Geometry: see drawing. Coordinates: mm, zero at the bounding-box minimum. Give positions to 0.01 mm unless a question says otherwise; leave off trailing zeros. Order: outer loops, then holes, each group sorted by start corner. A loop starts at its lowest first (then second) coordinate and runs counter-clockwise, first axis right, second up. Notation, with made-up numbers: M 79.5,37.25 L 109.5,37.25 A22 cw 109.5,56.25 Z; hole C 1,67.5 d4. An arc over 180 degrees is marked long. Use a Markdown table: item, result.
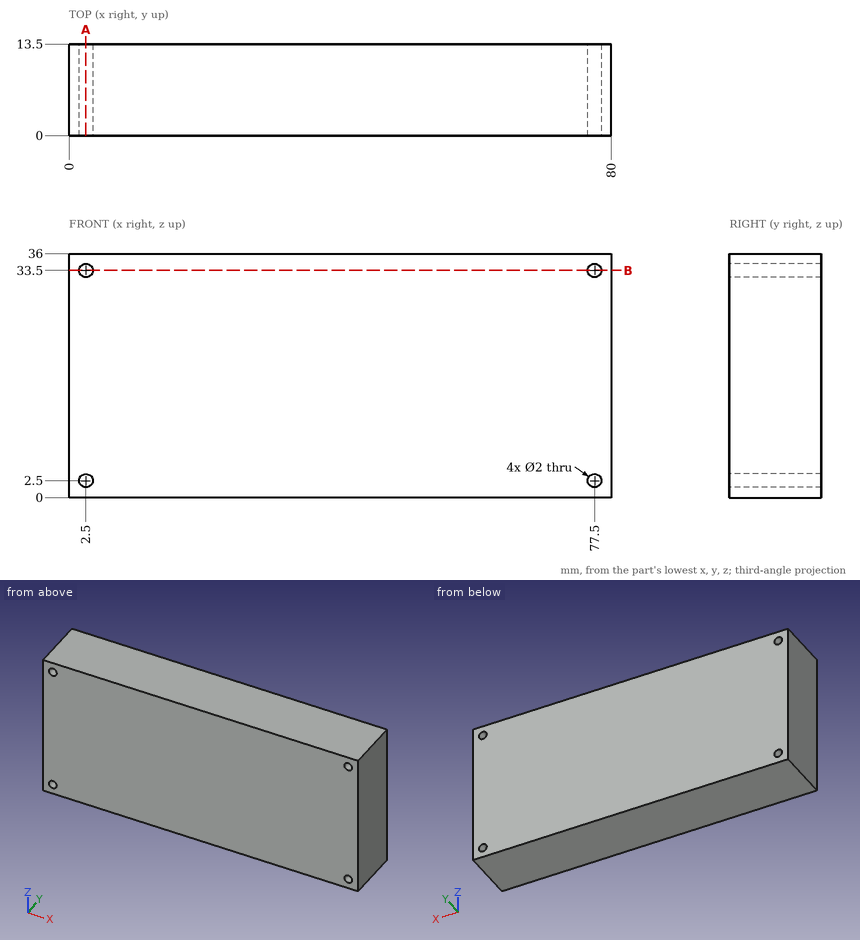
1) First-contact query: pin 1 Ø1.5 at (x, y) = (39, 9) entering from -Z; pin 2 Ø1.8 at (x, z) = (2.5, 33.5) entering from +Y. Flat tips, straight axial feed; report the tip coordinate or a pass-through.
Response values:
| item | result |
|---|---|
| pin 1 | stops at z = 0 |
| pin 2 | passes through |
2) Cut plane A-A on x = 2.5. Return loops of the section in (y, z).
Response values:
| item | result |
|---|---|
| outline | M 0,0 L 13.5,0 L 13.5,1.5 L 0,1.5 Z; M 0,3.5 L 13.5,3.5 L 13.5,32.5 L 0,32.5 Z; M 0,34.5 L 13.5,34.5 L 13.5,36 L 0,36 Z |
3) Material intervals for line 1 (Z direction, x = 2.5, y = 6.25); line 2 (X direction, y = 5.75, z = 33), sorted ascending. Write a range as from..to.
Response values:
| item | result |
|---|---|
| line 1 | z = 0..1.5, 3.5..32.5, 34.5..36 |
| line 2 | x = 0..1.63, 3.37..76.63, 78.37..80 |
4) Cut plane B-B on z = 33.5. Return loops of the section in (x, y).
Response values:
| item | result |
|---|---|
| outline | M 0,0 L 1.5,0 L 1.5,13.5 L 0,13.5 Z; M 3.5,0 L 76.5,0 L 76.5,13.5 L 3.5,13.5 Z; M 78.5,0 L 80,0 L 80,13.5 L 78.5,13.5 Z |
